Read the model definition and answer for the solid it produces. Units are mm, in the model's axes. Give positions to 0.01 mm unless a question says otherwise; leave off trailing zeros. Loops run counter-clockwise (first coordinate to the right, second up) from the corner with the lowest first, then second, coordinate; pieces in that order, holes last. Notation, with made-up numbers: (56.5, 71.25) - (98.5, 71.25) arc R32 cw to (98.5, 106.25) - close; hole circle Ø6 at (-22.75, 2). An arc over 180 degrees is marked (long way). Write item = value, one per line.
Autodesk Inventor part; units mm, degrees
ref_plane "YZ Plane" through (0, 0, 0) normal (1, 0, 0) x (0, 1, 0)
ref_plane "XZ Plane" through (0, 0, 0) normal (0, 1, 0) x (-1, 0, 0)
ref_plane "XY Plane" through (0, 0, 0) normal (0, 0, 1) x (1, 0, 0)
sketch "Sketch1" plane through (0, 0, 0) normal (0, 0, 1) x (1, 0, 0)
  line L0 (112.7125, -127) -> (-112.7125, -127)
  line L1 (-112.7125, -127) -> (-112.7125, 127)
  line L2 (-112.7125, 127) -> (112.7125, 127)
  line L3 (112.7125, 127) -> (112.7125, -127)
  line L4 (112.7125, -127) -> (-112.7125, 127) construction
  line L5 (-112.7125, -127) -> (112.7125, 127) construction
  point P0 (0, 0)
  dimension "d1" = 225.425
  dimension "d2" = 254
extrude "Plate1" add sketch "Sketch1" along normal blind 4.7625
sketch "Sketch2" plane through (0, 0, 4.7625) normal (0, 0, 1) x (1, 0, 0)
  line L0 (-69.85, 56.3563) -> (69.85, 56.3563)
  line L1 (69.85, 56.3563) -> (69.85, -56.3563)
  line L2 (69.85, -56.3563) -> (-69.85, -56.3563)
  line L3 (-69.85, -56.3563) -> (-69.85, 56.3563)
  line L4 (-69.85, 56.3563) -> (69.85, -56.3563) construction
  line L5 (69.85, 56.3563) -> (-69.85, -56.3563) construction
  point P0 (0, 0)
  dimension "d3" = 139.7
  dimension "d4" = 112.7125
extrude "Cut1" cut sketch "Sketch2" against normal blind 4.7625
equation "\"d5\" = Thickness"
equation "\"BendRadius\" = Thickness"
equation "\"BendReliefWidth\" = Thickness"
equation "\"BendReliefDepth\" = 0.5 * Thickness"
equation "\"CornerReliefSize\" = 4 * Thickness"
equation "\"MinimumRemnant\" = 2 * Thickness"
equation "\"TransitionRadius\" = BendRadius"
equation "\"JacobiRadiusSize\" = BendRadius"
equation "\"GapSize\" = Thickness"
equation "\"d0\" = BendRadius"
properties part number "LeftSide" material "Steel, Mild"
1) A cutting plane is placed at A-A on x = 63. Determine the outline of the cut face in (y, z), then the cut area to 3 significant figures.
Output:
outline = (-127, 0) - (-56.36, 0) - (-56.36, 4.76) - (-127, 4.76) - close; (56.36, 0) - (127, 0) - (127, 4.76) - (56.36, 4.76) - close
area = 673 mm²
2) A cutting plane is placed at C-C on z = 2.8. Determine the outline of the cut face in (x, y).
Output:
outline = (-112.71, -127) - (112.71, -127) - (112.71, 127) - (-112.71, 127) - close; hole (-69.85, -56.36) - (69.85, -56.36) - (69.85, 56.36) - (-69.85, 56.36) - close
3) A cutting plane is placed at B-B on y = 32. Determine the outline of the cut face in (x, z).
Output:
outline = (-112.71, 0) - (-69.85, 0) - (-69.85, 4.76) - (-112.71, 4.76) - close; (69.85, 0) - (112.71, 0) - (112.71, 4.76) - (69.85, 4.76) - close
4) Find the intervals of material crossed by probe 1 along Y at (x, z) = (61, 1.7); probe 2 along X at (y, z) = (-6.5, 2.3), in increasing order.
Output:
probe_1 = -127 to -56.36, 56.36 to 127
probe_2 = -112.71 to -69.85, 69.85 to 112.71
